from build123d import *

# Parameters (mm, degrees)
SKETCH2_W                    = 15
SKETCH2_H                    = 13
BOSS_EXTRUDE1_DEPTH          = 30
SKETCH3_W                    = 1
SKETCH3_H                    = 4
BOSS_EXTRUDE2_DEPTH          = 1
SKETCH4_R                    = 4
CUT_EXTRUDE3_DEPTH           = 22
SKETCH5_R                    = 2
CUT_EXTRUDE4_DEPTH           = 5
SKETCH7_R                    = 1.5
CUT_EXTRUDE5_DEPTH           = 30.706901555
FILLET4_R                    = 3
FILLET5_R                    = 3
F_8_0_3_DIAMETER_HOLE1_D     = 3
F_8_0_3_DIAMETER_HOLE1_DEPTH = 1.5


with BuildPart() as part:
    # Sketch2 → Boss-Extrude1 (new body)
    with BuildSketch(Plane(origin=(0, 0, 0), x_dir=(1, 0, 0), z_dir=(0, 1, 0))):
        Rectangle(SKETCH2_W, SKETCH2_H)
    extrude(amount=BOSS_EXTRUDE1_DEPTH)

    # Sketch3 → Boss-Extrude2 (add)
    with BuildSketch(Plane(origin=(0, 30, 0), x_dir=(1, 0, 0), z_dir=(0, 1, 0))):
        with Locations((7, 4.5)):
            Rectangle(SKETCH3_W, SKETCH3_H)
        with Locations((7, -4.5)):
            Rectangle(SKETCH3_W, SKETCH3_H)
        with Locations((-7, -4.5)):
            Rectangle(SKETCH3_W, SKETCH3_H)
        with Locations((-7, 4.5)):
            Rectangle(SKETCH3_W, SKETCH3_H)
    extrude(amount=BOSS_EXTRUDE2_DEPTH)

    # Sketch4 → Cut-Extrude3 (cut)
    with BuildSketch(Plane(origin=(0, 30, 0), x_dir=(1, 0, 0), z_dir=(0, 1, 0))):
        with Locations(Location((0, 0, 0), (0, 0, 270))):
            Circle(SKETCH4_R)
    extrude(amount=-CUT_EXTRUDE3_DEPTH, mode=Mode.SUBTRACT)

    # Sketch5 → Cut-Extrude4 (cut)
    with BuildSketch(Plane(origin=(0, 8, 0), x_dir=(1, 0, 0), z_dir=(0, 1, 0))):
        with Locations(Location((0, 0, 0), (0, 0, 270))):
            Circle(SKETCH5_R)
    extrude(amount=-CUT_EXTRUDE4_DEPTH, mode=Mode.SUBTRACT)

    # Sketch7 → Cut-Extrude5 (cut, through all)
    with BuildSketch(Plane(origin=(0, 3, 0), x_dir=(1, 0, 0), z_dir=(0, 1, 0))):
        with Locations(Location((0, 0, 0), (0, 0, 270))):
            Circle(SKETCH7_R)
    extrude(amount=-CUT_EXTRUDE5_DEPTH, mode=Mode.SUBTRACT)

    # Fillet4
    # the kernel refuses this fillet: 3 mm, written as the material it takes off along each edge
    with BuildSketch(Plane(origin=(0, 8, 0), x_dir=(0, 0, 1), z_dir=(-1, 0, 0))) as fillet4_piece_1:
        with BuildLine():
            CenterArc((5, -2.828427125), FILLET4_R, 109.471220634, 70.528779366)
            Line((2, -2.828427125), (1.94, -2.828427125))
            Line((1.94, -2.828427125), (1.94, 0))
            Line((1.94, 0), (2, 0.06))
            ThreePointArc((2, 0.06), (3, 0.06), (3.98, 0.056568542))
            Line((3.98, 0.056568542), (4, 0))
        make_face()
    revolve(axis=Axis((0, 8, 0), (0, 1, 0)), mode=Mode.SUBTRACT)

    # Fillet5
    # the kernel refuses this fillet: 3 mm, written as the material it takes off along each edge
    with BuildSketch(Plane(origin=(0, 3, 0), x_dir=(0, 0, 1), z_dir=(-1, 0, 0))) as fillet5_piece_1:
        with BuildLine():
            CenterArc((4.5, -1.658312395), FILLET5_R, 146.442690238, 33.557309762)
            Line((2, 0), (1.95, 0.033166248))
            ThreePointArc((1.95, 0.033166248), (1.75, 0.06), (1.5, 0.06))
            Line((1.5, 0.06), (1.44, 0))
            Line((1.44, 0), (1.44, -1.658312395))
            Line((1.44, -1.658312395), (1.5, -1.658312395))
        make_face()
    revolve(axis=Axis((0, 3, 0), (0, 1, 0)), mode=Mode.SUBTRACT)

    # Ø8.0 (3) Diameter Hole1
    with Locations(Plane(origin=(7.5, 7, 0), x_dir=(0, 0, 1), z_dir=(1, 0, 0))):
        with Locations((0, 0), (0, -16)):
            Hole(F_8_0_3_DIAMETER_HOLE1_D / 2, depth=F_8_0_3_DIAMETER_HOLE1_DEPTH)


solid = part.part
Geometry: final body of the model. Coordinates: model frame, mm. A direction names the side the tool comes from. Coordinates: 2 decimals unless noted, no trailing zeros. Order: outer loops, then holes, each group sorted by start corner. A loop starts at its lowest first (then second) coordinate and runs counter-clockwise, first axis right, second up. Notation, with made-up numbers: M 68.25,12.5 L 85.25,12.5 A26 ccw 85.25,39.5 Z; hole C 17.5,-0.75 d1. An arc over 180 degrees is marked long. One line per question, with ' | ' between items. Start each with the question number.
Item 1: Cut plane A-A, the plane z = 0. Return the cut outline in (x, y), then the cut area to 3 significant figures.
Item 2: Draft query along X for faces 1 (the flat face through (6, 23, 0)), 2 (the flat face through (0, 0, -2)), 3 (the cylindrical face through (0.45, 0.68, 1.43)). Return one class per face: released by +X, released by -X, zero draft, split by the parting line, or undercut.
Item 3: Ray query, probe 1 along Y at (x, z) = (7.2, 0); probe 2 along X at (y, z) = (21.75, 0); probe 3 along X at (y, z) = (20.5, 0). Return the intervals inside material, ascending. Write a range as [from, to].
Item 4: Cut plane C-C, the plane y = 23. Return the cut outline in (x, z), then the cut area to 3 significant figures.
Item 5: Cut plane B-B, the plane x = 0. Return the cut outline in (y, z).
Item 6: Set-up query: faces 4 (the flat face through (-6.5, 30.5, 4.5)), 5 (the flat face through (-7, 30.5, 2.5)), 6 (the cylindrical face through (-3.905, 19.154, -0.867)). Return all of +Z, -Z, +X, -X, +Y, -Y with unobstructed straight access to the full face (end or side cutting, diameter ignored); none if empty.
Item 7: Pin query (flat end, axial travel): pin 1 Ø3 at (x, z) = (3.5, -4.5) entering from +Y; pin 2 Ø6.5 at (x, z) = (0, 0) entering from +Y; pin 3 Ø3.5 at (x, z) = (0, 0) entering from +Y. Return the tip coordinate at first contact, or that it passes through.
Item 8: Cut plane D-D, the plane z = 5.25. Return the cut outline in (x, y).
A:
1) outline: M -7.5,0 L -1.5,0 L -1.5,1.34 A3 ccw -2,3 L -2,5.17 A3 ccw -4,8 L -4,30 L -7.5,30 Z; M 1.5,0 L 7.5,0 L 7.5,5.5 L 6,5.5 L 6,8.5 L 7.5,8.5 L 7.5,21.5 L 6,21.5 L 6,24.5 L 7.5,24.5 L 7.5,30 L 4,30 L 4,8 A3 ccw 2,5.17 L 2,3 A3 ccw 1.5,1.34 Z | area: 232 mm2
2) face 1: released by +X | face 2: zero draft | face 3: undercut
3) probe 1: y = [0, 5.5], [8.5, 21.5], [24.5, 30] | probe 2: x = [-7.5, -4], [4, 6] | probe 3: x = [-7.5, -4], [4, 7.5]
4) outline: M -7.5,-6.5 L 7.5,-6.5 L 7.5,-1.5 L 6,-1.5 L 6,1.5 L 7.5,1.5 L 7.5,6.5 L -7.5,6.5 Z; hole C 0,0 d8 | area: 140 mm2
5) outline: M 0,-6.5 L 30,-6.5 L 30,-4 L 8,-4 A3 ccw 5.17,-2 L 3,-2 A3 ccw 1.34,-1.5 L 0,-1.5 Z; M 0,1.5 L 1.34,1.5 A3 ccw 3,2 L 5.17,2 A3 ccw 8,4 L 30,4 L 30,6.5 L 0,6.5 Z
6) face 4: +Z, -Z, +Y | face 5: +X, -X, +Y | face 6: +Y
7) pin 1: stops at y = 30 | pin 2: stops at y = 7.61 | pin 3: stops at y = 2.54
8) outline: M -7.5,0 L 7.5,0 L 7.5,31 L 6.5,31 L 6.5,30 L -6.5,30 L -6.5,31 L -7.5,31 Z
